from build123d import *

# Parameters (mm, degrees)
BOSS_EXTRUDE2_DEPTH = 2.97
SKETCH5_W           = 7.5
SKETCH5_H           = 2.83
BOSS_EXTRUDE3_DEPTH = 2.8


with BuildPart() as part:
    # Sketch3 → Boss-Extrude2 (new body)
    with BuildSketch(Plane.XY):
        with BuildLine():
            Line((-14.345, 4.51436853), (14.345, 4.51436853))
            ThreePointArc((14.345, 4.51436853), (18.85936853, 0), (14.345, -4.51436853))
            Line((14.345, -4.51436853), (-14.345, -4.51436853))
            ThreePointArc((-14.345, -4.51436853), (-18.85936853, 0), (-14.345, 4.51436853))
        make_face()
        with BuildLine():
            Line((-14.345, 0.84436853), (-9.035, 0.84436853))
            ThreePointArc((-9.035, 0.84436853), (-8.19063147, 0), (-9.035, -0.84436853))
            Line((-9.035, -0.84436853), (-14.345, -0.84436853))
            ThreePointArc((-14.345, -0.84436853), (-15.18936853, 0), (-14.345, 0.84436853))
        make_face(mode=Mode.SUBTRACT)
        with BuildLine():
            Line((14.345, -0.84436853), (9.035, -0.84436853))
            ThreePointArc((9.035, -0.84436853), (8.19063147, 0), (9.035, 0.84436853))
            Line((9.035, 0.84436853), (14.345, 0.84436853))
            ThreePointArc((14.345, 0.84436853), (15.18936853, 0), (14.345, -0.84436853))
        make_face(mode=Mode.SUBTRACT)
    extrude(amount=BOSS_EXTRUDE2_DEPTH)

    # Sketch5 → Boss-Extrude3 (add)
    with BuildSketch(Plane.XY.offset(2.97)):
        Rectangle(SKETCH5_W, SKETCH5_H)
    extrude(amount=BOSS_EXTRUDE3_DEPTH)


solid = part.part
Geometry: final body of the model. Coordinates: model frame, mm. A direction names the side the tool comes from. Round coordinates to 2 decimals unless told otherwise and drop trailing zeros. Order: outer loops, then holes, each group sorted by start corner. A loop starts at its lowest first (then second) coordinate and runs counter-clockwise, first axis right, second up. Notation, with made-up numbers: (42.5, 27.5) -> (91.5, 27.5) arc R33 ccw to (91.5, 57.5) -> close; hole circle Ø10 at (67, 10). An arc over 180 degrees is marked (long way). Put each result on its own line as item: value. Start each with the question number.
Q1. Section D-D on y = 2.5. Return the cut outline in (x, z).
Q2. Line query: probe 1 along X at (y, z) = (0, 0.95); probe 2 along Y at (x, z) = (12.5, 2); probe 3 along Z at (x, y) = (-9, 2.25). Output: solid intervals per line, ascending.
Q3. Section A-A on y = 0. Return the cut outline in (x, z), and give its area (3 significant figures).
Q4. Section C-C on z = 3.95. Return the cut outline in (x, y) (3 decimals), and give its area (3 significant figures).
Q5. First-contact query: pin 1 (0.8 mm diameter, centred on y = 0.5, z = 4, fed in from +X); pin 2 (0.8 mm diameter, centred on x = 0.5, z = 4, fed in from +Y) (3 decimals); pin 3 (2 mm diameter, centred on y = 0, z = 4, fed in from -X). Flat tips, straight axial feed; report the tip coordinate or a pass-through.
Q6. Pull-direction query (Y, two-part tool) for faces 1 (the flat face through (0, 1.415, 4)), 2 (the flat face through (-3.75, 0, 4)), 3 (the cylindrical face through (-15.19, -0.02, 1.46)); classes: +Y half, -Y half, draft (parallel to the pull), parting line (faces both ways), or undercut.
Q7. Section B-B on z = 1.45. Return the cut outline in (x, y) (3 decimals), and give its area (3 significant figures).
Q8. Reachability of faces 4 (the cylindrical face through (8.19, -0.02, 1.46)), 5 (the flat face through (3.75, 0, 4)), 6 (the flat face through (0, 0, 0)) from +Z, -Z, +X, -X, +Y, -Y: full face, straight path, thin tool, end or side. Return the list, or none.
Ans:
1. outline: (-18.1, 0) -> (18.1, 0) -> (18.1, 2.97) -> (-18.1, 2.97) -> close
2. probe 1: x = -18.86 to -15.19, -8.19 to 8.19, 15.19 to 18.86
2. probe 2: y = -4.51 to -0.84, 0.84 to 4.51
2. probe 3: z = 0 to 2.97
3. outline: (-18.86, 0) -> (-15.19, 0) -> (-15.19, 2.97) -> (-18.86, 2.97) -> close; (-8.19, 0) -> (8.19, 0) -> (8.19, 2.97) -> (3.75, 2.97) -> (3.75, 5.77) -> (-3.75, 5.77) -> (-3.75, 2.97) -> (-8.19, 2.97) -> close; (15.19, 0) -> (18.86, 0) -> (18.86, 2.97) -> (15.19, 2.97) -> close
3. area: 91.5 mm2
4. outline: (-3.75, -1.415) -> (3.75, -1.415) -> (3.75, 1.415) -> (-3.75, 1.415) -> close
4. area: 21.2 mm2
5. pin 1: stops at x = 3.75
5. pin 2: stops at y = 1.415
5. pin 3: stops at x = -3.75
6. face 1: +Y half
6. face 2: draft
6. face 3: undercut
7. outline: (-14.345, -4.514) -> (14.345, -4.514) arc R4.514 ccw to (14.345, 4.514) -> (-14.345, 4.514) arc R4.514 ccw to start; hole (-14.345, -0.844) -> (-9.035, -0.844) arc R0.844 ccw to (-9.035, 0.844) -> (-14.345, 0.844) arc R0.844 ccw to start; hole (9.035, -0.844) -> (14.345, -0.844) arc R0.844 ccw to (14.345, 0.844) -> (9.035, 0.844) arc R0.844 ccw to start
7. area: 301 mm2
8. face 4: +Z, -Z
8. face 5: +Z, +X, +Y, -Y
8. face 6: -Z, +X, -X, +Y, -Y
